```python
from build123d import *

# Parameters (mm, degrees)
F0_W     = 40
F0_H     = 5
F1_DEPTH = 1
F3_DEPTH = 71
F4_W     = 0.4
F4_H     = 0.2
F5_DEPTH = 40.001


with BuildPart() as f1:
    # F0 (on Top) → F1 (new body)
    with BuildSketch(Plane.XY):
        Rectangle(F0_W, F0_H)
    extrude(amount=F1_DEPTH)

    # F2 (on Top) → F3 (join)
    with BuildSketch(Plane.XY):
        Polygon((-15.669873, 0), (-20, 2.5), (-20, -2.5), align=None)
        Polygon((20, 0), (15.669873, 2.5), (15.669873, -2.5), align=None)
    extrude(amount=F3_DEPTH)

    # F4 (on face) → F5 (cut, through all)
    with BuildSketch(Plane(origin=(-20, 0, 0), x_dir=(0, -1, 0), z_dir=(-1, 0, 0))):
        with Locations((2.3, 11.1)):
            Rectangle(F4_W, F4_H)
        with Locations((2.3, 21.1)):
            Rectangle(F4_W, F4_H)
        with Locations((2.3, 31.1)):
            Rectangle(F4_W, F4_H)
        with Locations((2.3, 41.1)):
            Rectangle(F4_W, F4_H)
        with Locations((2.3, 51.1)):
            Rectangle(F4_W, F4_H)
        with Locations((2.3, 61.1)):
            Rectangle(F4_W, F4_H)
        with Locations((2.3, 71.1)):
            Rectangle(F4_W, F4_H)
    extrude(amount=-F5_DEPTH, mode=Mode.SUBTRACT)


solid = f1.part
```
Work out the finished part from the listing and answer in its coordinate system (mm). A direction names the side the tool comes from. Give positions to 0.01 mm unless a question says otherwise; leave off trailing zeros. Order: outer loops, then holes, each group sorted by start corner. A loop starts at its lowest first (then second) coordinate and runs counter-clockwise, first axis right, second up. Notation, with made-up numbers: M 54.25,35 L 91.25,35 A15 ccw 91.25,56 Z; hole C -12.75,48 d5. An arc over 180 degrees is marked long. Return JSON: item names as keys, results as strings.
1) Straight lines are drawn through the part: line 1 along Z through (x, y) = (14, -0.8); line 2 along X through (y, z) = (-1.15, 35); line 3 along X through (y, z) = (-0.9, 15). For each, find the intervals that lie inside material, in ascending order. Write a range as [from, to].
Resolved:
{"line 1": "[0, 1]", "line 2": "[-20, -17.66], [15.67, 18.01]", "line 3": "[-20, -17.23], [15.67, 18.44]"}
2) A tool of negligible diameter and unlimited length cuts with its end or side. For faces 1 (the flat face through (15.67, 0, 36)), 2 (the flat face through (19, -2, 1)), 3 (the flat face through (-17.8, 1.23, 35.51)), 4 (the flat face through (17.87, 1.23, 35.51)), from which of +Z, -Z, +X, -X, +Y, -Y can it reach the whole face along a straight path? Write none if from no direction.
Resolved:
{"face 1": "+Z, +Y, -Y", "face 2": "+Z, +X, -Y", "face 3": "+Z, +Y", "face 4": "+Z, +X, +Y"}
3) Section C-C, the plane x = -3 is taken. Write down the section's boundary in (y, z).
Resolved:
{"outline": "M -2.5,0 L 2.5,0 L 2.5,1 L -2.5,1 Z"}
4) Section A-A, the plane z = 28 is taken. Write down the section's boundary in (x, y).
Resolved:
{"outline": "M -20,-2.5 L -15.67,0 L -20,2.5 Z; M 15.67,-2.5 L 20,0 L 15.67,2.5 Z"}
5) Each of these flat-tipped pins is pushed along its axis until it touches: pin 1 (3 mm diameter, centred on x = -8, y = 1.5, fed in from +Z); pin 2 (1 mm diameter, centred on y = 1.5, z = 57.5, fed in from +X). Where does it stop, or does it pass through?
Resolved:
{"pin 1": "z = 1", "pin 2": "x = 18.27"}
6) Section B-B, the plane y = -1.05 is taken. Write down the section's boundary in (x, z).
Resolved:
{"outline": "M -20,0 L 20,0 L 20,1 L 18.18,1 L 18.18,71 L 15.67,71 L 15.67,1 L -17.49,1 L -17.49,71 L -20,71 Z"}
7) For a pull along X with two mould halves and no side action, classify faces 5 (the flat face through (17.8, -1.27, 35.51)), 6 (the flat face through (-17.87, -1.27, 35.51)), 7 (the flat face through (0, 0, 0)) as +X half, -X half, draft (parallel to the pull), parting line (faces both ways), or undercut.
Resolved:
{"face 5": "+X half", "face 6": "undercut", "face 7": "draft"}
